Can you work these out from the model? Positions are in its coordinate system, mm. A direction names the side the tool comes from. Coordinates: 2 decimals unless noted, no trailing zeros. Order: outer loops, then holes, each group sorted by start corner. A loop starts at its lowest first (then second) coordinate and runs counter-clockwise, first axis right, second up. Notation, with made-up numbers: (50.25, 10.25) -> (64.25, 10.25) arc R17 ccw to (64.25, 38.25) -> close; hole circle Ø4 at (-39, 0.5). An arc over 180 degrees is marked (long way). Return JSON: item names as keys, results as strings. Group by question number.
1) For pin 1 (2.5 mm diameter, centred on x = -15.5, z = 15.5, fed in from +Y), with a flat end and sliding along its axis, tell me the tip position at first contact or that it passes through.
2) If we section it at B-B, the plane x = 0: Please give me the cut outline in (y, z).
3) Thinking about a two-plate mould opening in X: for faces 3 (the cylindrical face through (17.287, 1.521, -17.248)), 4 (the cylindrical face through (13.926, 1.479, 15.004)), 5 (the flat face through (16.1, 3, -7.9)), which applies, +X half, -X half, draft (parallel to the pull), parting line (faces both ways), or undercut?
4) If I drill on probe 1 along Z at (x, y) = (-15.5, 0.85); probe 2 along X at (y, z) = (0.5, 0); probe 3 along X at (y, z) = (2.1, 0), over which ranges is the centre line in solid material (lowest first)? Write a range as from..to.
5) If we section it at C-C, the plane y = 1.1: Please give me the cut outline in (x, z).
6) If we section it at D-D, the plane x = -15: Please give me the cut outline in (y, z).
7) If we section it at A-A, the plane z = 0: Please give me the cut outline in (x, y).
8) For faces 1 (the cylindrical face through (17.328, 2.392, -3.848)), 2 (the cylindrical face through (-17.287, 1.521, 17.248)), which set-ups out of +Z, -Z, +X, -X, +Y, -Y let a thin tool reach every point of the face, with its end or its side?
Autodesk Inventor part; units mm, degrees
ref_plane "YZ Plane" through (0, 0, 0) normal (1, 0, 0) x (0, 1, 0)
ref_plane "XZ Plane" through (0, 0, 0) normal (0, 1, 0) x (-1, 0, 0)
ref_plane "XY Plane" through (0, 0, 0) normal (0, 0, 1) x (1, 0, 0)
sketch "Sketch1" plane through (0, 0, 0) normal (0, 1, 0) x (-1, 0, 0)
  line L0 (-18, 18) -> (18, 18)
  line L1 (18, 18) -> (18, -18)
  line L2 (18, -18) -> (-18, -18)
  line L3 (-18, -18) -> (-18, 18)
  line L4 (-18, 18) -> (18, -18) construction
  line L5 (18, 18) -> (-18, -18) construction
  circle A0 centre (15.5, -15.5) radius 1.65
  circle A1 centre (15.5, 15.5) radius 1.65
  circle A2 centre (-15.5, 15.5) radius 1.65
  circle A3 centre (-15.5, -15.5) radius 1.65
  circle A4 centre (0, 0) radius 14
  dimension "d0" = 36
  dimension "d1" = 36
  dimension "d2" = 3.3
  dimension "d3" = 3.3
  dimension "d4" = 3.3
  dimension "d5" = 3.3
  dimension "d6" = 2.5
  dimension "d7" = 2.5
  dimension "d8" = 2.5
  dimension "d9" = 2.5
  dimension "d10" = 28
extrude "Extrusion1" add sketch "Sketch1" along normal blind 3
fillet "Fillet1" radius 2.5 4 edges at (-18, 1.5, 18) (18, 1.5, 18) (18, 1.5, -18) (-18, 1.5, -18)
sketch "Sketch2" plane through (0, 3, 0) normal (0, 1, 0) x (1, 0, 0)
  circle A0 centre (0, 0) radius 14
hole "Hole1" at (0, 3, 0) direction (0, -1, 0) diameter 35.5 depth 1.2
properties part number "Bearing Block P2" material "Aluminum 6061"
Result sheet:
{
 "1": {"pin 1": "passes through"},
 "2": {"outline": "(0, -18) -> (3, -18) -> (3, -17.75) -> (1.8, -17.75) -> (1.8, -14) -> (0, -14) -> close; (0, 14) -> (1.8, 14) -> (1.8, 17.75) -> (3, 17.75) -> (3, 18) -> (0, 18) -> close"},
 "3": {"face 3": "+X half", "face 4": "undercut", "face 5": "draft"},
 "4": {"probe 1": "z = -18..-17.15, -13.85..13.85, 17.15..18", "probe 2": "x = -18..-14, 14..18", "probe 3": "x = -18..-17.75, 17.75..18"},
 "5": {"outline": "(-18, -15.5) arc R2.5 ccw to (-15.5, -18) -> (15.5, -18) arc R2.5 ccw to (18, -15.5) -> (18, 15.5) arc R2.5 ccw to (15.5, 18) -> (-15.5, 18) arc R2.5 ccw to (-18, 15.5) -> close; hole circle Ø3.3 at (-15.5, -15.5); hole circle Ø3.3 at (-15.5, 15.5); hole circle Ø28 at (0, 0); hole circle Ø3.3 at (15.5, -15.5); hole circle Ø3.3 at (15.5, 15.5)"},
 "6": {"outline": "(0, -18) -> (3, -18) -> (3, -17.07) -> (0, -17.07) -> close; (0, -13.93) -> (3, -13.93) -> (3, -9.49) -> (1.8, -9.49) -> (1.8, 9.49) -> (3, 9.49) -> (3, 13.93) -> (0, 13.93) -> close; (0, 17.07) -> (3, 17.07) -> (3, 18) -> (0, 18) -> close"},
 "7": {"outline": "(-18, 0) -> (-14, 0) -> (-14, 1.8) -> (-17.75, 1.8) -> (-17.75, 3) -> (-18, 3) -> close; (14, 0) -> (18, 0) -> (18, 3) -> (17.75, 3) -> (17.75, 1.8) -> (14, 1.8) -> close"},
 "8": {"face 1": "+Y", "face 2": "+Z, -X, +Y, -Y"}
}
